Autodesk Inventor part; units mm, degrees
ref_plane "YZ Plane" through (0, 0, 0) normal (1, 0, 0) x (0, 1, 0)
ref_plane "XZ Plane" through (0, 0, 0) normal (0, 1, 0) x (-1, 0, 0)
ref_plane "XY Plane" through (0, 0, 0) normal (0, 0, 1) x (1, 0, 0)
sketch "Sketch1" plane through (0, 0, 0) normal (0, 0, 1) x (1, 0, 0)
  line L0 (-44.6809, 2.5) -> (-7.5647, 2.5)
  line L1 (-44.6809, 0) -> (-44.6809, 2.5)
  line L2 (0, 0) -> (0, 19.2246)
  arc A0 (-3.8253, -1.3563) -> (-6.7141, 3.5099) centre (0, 4.2052) ccw
  arc A1 (-2.5687, 0.8193) -> (-4.0285, 2.8511) centre (0, 4.2052) ccw
  arc A2 (-2.5687, 0.8193) -> (-7.5647, 2.5) centre (-7.5647, -5.7659) ccw
  line L3 (-4.0285, 2.8511) -> (-6.7141, 3.5099)
  arc A3 (-3.8253, -1.3563) -> (-8.1904, 0) centre (-8.1904, -7.7027) ccw
  line L4 (-8.1904, 0) -> (-44.6809, 0)
  line L5 (-36.0171, 0) -> (-5.5909, 0)
  line L6 (-5.2801, 0) -> (0, 0)
  point P0 (0, 10.9552)
  point P1 (0, 8.4552)
  dimension "d1" = 2.5
  dimension "d2" = 2.5
  dimension "d3" = 8.5
extrude "Extrusion1" add sketch "Sketch1" along normal mid plane 100 contours L0 A2 A1 L2 A0 A3 L4 L1 | A1 L3 A0 L2
sketch "Sketch2" plane through (-44.6809, 2.5, 50) normal (0, 1, 0) x (1, 0, 0)
  circle A0 centre (20, 90) radius 4
  circle A1 centre (10, 50) radius 4
  circle A2 centre (20, 10) radius 4
  line L0 (0, 100) -> (37.1161, 100)
  line L1 (0, 100) -> (0, 0)
  line L2 (37.1161, 0) -> (0, 0)
  point P0 (44.6809, 50)
  dimension "d6" = 8
  dimension "d7" = 8
  dimension "d8" = 8
  dimension "d9" = 10
  dimension "d10" = 20
  dimension "d11" = 20
  dimension "d12" = 10
  dimension "d13" = 10
  dimension "d14" = 50
extrude "Extrusion2" cut sketch "Sketch2" against normal up to next draft -20
sketch "Sketch4" plane through (-44.6809, 2.5, 50) normal (0, 1, 0) x (1, 0, 0)
  line L0 (36.4904, 100) -> (36.4904, 0)
  line L1 (36.4904, 80) -> (67.1636, 80)
  line L2 (67.1636, 80) -> (67.1636, 60)
  line L3 (67.1636, 60) -> (36.4904, 60)
  line L4 (36.4904, 60) -> (36.4904, 80)
  line L5 (36.4904, 40) -> (70.3914, 40)
  line L6 (70.3914, 40) -> (70.3914, 20)
  line L7 (70.3914, 20) -> (36.4904, 20)
  line L8 (36.4904, 20) -> (36.4904, 40)
  line L9 (37.1161, 0) -> (0, 0)
  line L10 (51.4309, 100) -> (37.9309, 100)
  point P0 (44.6809, 50)
  point P1 (37.9668, 100)
  point P2 (40.8556, 100)
  dimension "d22" = 20
  dimension "d23" = 20
  dimension "d24" = 20
  dimension "d25" = 20
extrude "Extrusion3" cut sketch "Sketch4" against normal mid plane 100
properties part number "Hinge1" material "Stainless Steel"
Part model, mm, in its own coordinate system. A direction names the side the tool comes from. Give positions to 0.01 mm unless a question says otherwise; leave off trailing zeros. Order: outer loops, then holes, each group sorted by start corner. A loop starts at its lowest first (then second) coordinate and runs counter-clockwise, first axis right, second up. Notation, with made-up numbers: (76, 60) - (96, 60) arc R13 cw to (96, 72) - close; hole circle Ø8 at (13, -20.5). An arc over 180 degrees is marked (long way). One line per question, with ' | ' between items.
1. Band-saw the part on D-D on x = -23. Give the number of separate pieces and of enclosed holes in the cut face, then the cut area to 3 significant figures.
Filled in:
separate pieces: 3 | enclosed holes: 0 | area: 219 mm²
2. Band-saw the part on A-A on z = -40. List the corners of the cut face in (x, y), then the cut area to 3 significant figures.
Filled in:
outline: (-44.68, 0) - (-27.77, 0) - (-28.68, 2.5) - (-44.68, 2.5) - close; (-21.59, 0) - (-8.19, 0) arc R7.7 cw to (-3.83, -1.36) arc R6.75 ccw (long way) to (-6.71, 3.51) - (-4.03, 2.85) arc R4.25 cw (long way) to (-2.57, 0.82) arc R8.27 ccw to (-7.56, 2.5) - (-20.68, 2.5) - close | area: 163 mm²
3. Band-saw the part on B-B on y = 10. List the corners of the cut face in (x, z), then the cut area to 3 significant figures.
Filled in:
outline: (-3.46, -50) - (3.46, -50) - (3.46, -30) - (-3.46, -30) - close; (-3.46, -10) - (3.46, -10) - (3.46, 10) - (-3.46, 10) - close; (-3.46, 30) - (3.46, 30) - (3.46, 50) - (-3.46, 50) - close | area: 415 mm²
4. Band-saw the part on C-C on z = 32. List the corners of the cut face in (x, y), then the cut area to 3 significant figures.
Filled in:
outline: (-44.68, 0) - (-8.19, 0) arc R7.7 cw to (-3.83, -1.36) arc R6.75 ccw (long way) to (-6.71, 3.51) - (-4.03, 2.85) arc R4.25 cw (long way) to (-2.57, 0.82) arc R8.27 ccw to (-7.56, 2.5) - (-44.68, 2.5) - close | area: 181 mm²
5. Drill centre lines: probe 1 along Z at (x, y) = (-5, 1.5); probe 2 along Y at (x, z) = (-14.5, -40); probe 3 along X at (y, z) = (0.75, -40). Where is each one in solid material? Low to high.
Filled in:
probe 1: -50 to -30, -10 to 10, 30 to 50 | probe 2: 0 to 2.5 | probe 3: -44.68 to -28.04, -21.32 to -2.47, 2.47 to 5.8
6. Drop flat-ended pins along their axis: P1, Ø2, axis at y = 1.5, z = 15.5, coming from the +X side; P2, Ø10, axis at x = -26, z = 32, coming from the -Y side; P3, Ø10, axis at x = -5, z = -29, coming from the -Y side. Give the stop position or say it passes through.
Filled in:
P1: x = -8.19 | P2: y = 0 | P3: y = -2.54
7. Pull direction Y, two halves, no side cores. Call faces 1 (the face through (-44.681, 1, -1)), 2 (the face through (-5.936, -0.337, 39.86)), 3 (the face through (-4.96, 2.08, -0.14)): +Y half, -Y half, draft (parallel to the pull), parting line (faces both ways), or undercut.
Filled in:
face 1: draft | face 2: -Y half | face 3: undercut
8. Which spindle directions (+Z, -Z, +X, -X, +Y, -Y) get a long thin tool onto all of the face, cutting with end or side? Do faces 4 (the face through (-5.353, 3.176, 39.86)), 5 (the face through (-26, 0, -1)), 6 (the face through (-21.774, 0.156, -38.795)), 7 (the face through (-4.96, 2.08, -40.14)), 8 (the face through (-4.14, 5.8, 10)). Say none if no direction does.
Filled in:
face 4: +Z, -Z, -X | face 5: +Z, -Z, -X, -Y | face 6: +Y | face 7: +Z, -Z | face 8: +X, +Y, -Y
